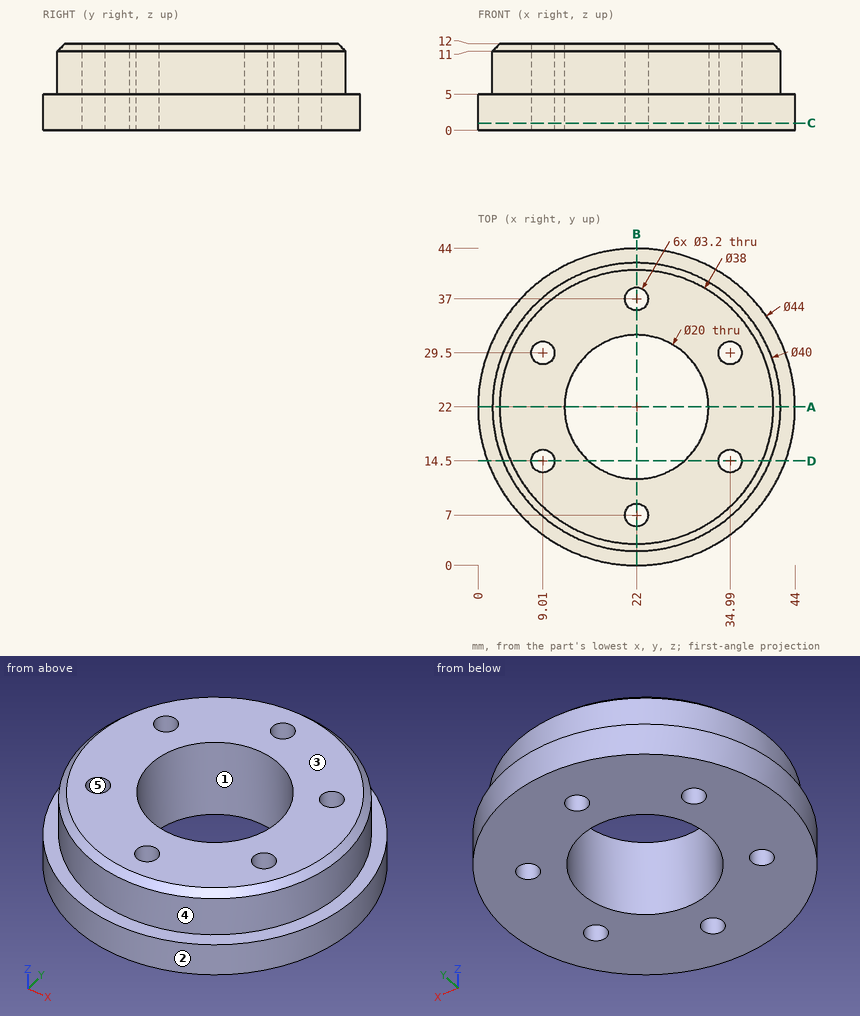
Job drawing, mm, ordinate dimensions from the low corner. One solid piece. A direction names the side the tool comes from. Round coordinates to 2 decimals unless told otherwise and drop trailing zeros. Write each loop counter-clockwise with the first axis right and the second up, starting at its lowest first coordinate (ties: lowest second). Pieces come first, ordered by that corner, then holes.
1) Mould opens along X. For the marked faces 1, 2 and 3 say: +X half, -X half, draft (parallel to the pull), parting line (faces both ways), or undercut.
2) Pin check, flat tips, straight feed: pin 1 (6 mm diameter, centred on y = 14, z = 9, fed in from +X) (1 decimal); pin 2 (3.5 mm diameter, centred on x = 34.99, y = 29.5, fed in from +Z); pin 3 (1 mm diameter, centred on y = 30.5, z = 10.5, fed in from -X); pin 4 (1.5 mm diameter, centred on y = 38, z = 10.5, fed in from -X). Stop position of each tip, or through.
3) 3-axis set-ups, long thin cutter, end or side, ignore diameter. For the marked faces 4 and 5: which of +Z, -Z, +X, -X, +Y, -Y reach the whole face in a straight line?
4) Band-saw the part on C-C, the plane z = 1. List the corners of the cut face in (x, y), and give its area (3 significant figures).
5) Band-saw the part on D-D, the plane y = 14.5. Give the number of separate pieces and of enclosed holes in the cut face, and give its area (3 significant figures).
6) Drill centre lines: probe 1 along Y at (x, z) = (22, 5.5); probe 2 along X at (y, z) = (29.5, 5.5) (1 decimal); probe 3 along Y at (x, z) = (10, 7.75) (1 decimal). Where is each one in solid material? Low to high.
7) Band-saw the part on A-A, the plane y = 22. List the corners of the cut face in (x, z), and give its area (3 significant figures).
8) Band-saw the part on B-B, the plane x = 22. List the corners of the cut face in (y, z).
Ans:
1. face 1: undercut
1. face 2: parting line
1. face 3: draft
2. pin 1: stops at x = 41.4
2. pin 2: stops at z = 12
2. pin 3: stops at x = 3.67
2. pin 4: stops at x = 9.06
3. face 4: +Z
3. face 5: +Z, -Z
4. outline: circle Ø44 at (22, 22); hole circle Ø3.2 at (9.01, 14.5); hole circle Ø3.2 at (9.01, 29.5); hole circle Ø20 at (22, 22); hole circle Ø3.2 at (22, 7); hole circle Ø3.2 at (22, 37); hole circle Ø3.2 at (34.99, 14.5); hole circle Ø3.2 at (34.99, 29.5)
4. area: 1,160 mm2
5. separate pieces: 4
5. enclosed holes: 0
5. area: 230 mm2
6. probe 1: y = 2 to 5.4, 8.6 to 12, 32 to 35.4, 38.6 to 42
6. probe 2: x = 3.5 to 7.4, 10.6 to 15.4, 28.6 to 33.4, 36.6 to 40.5
6. probe 3: y = 6 to 13.2, 15.8 to 28.2, 30.8 to 38
7. outline: (0, 0) - (12, 0) - (12, 12) - (3, 12) - (2, 11) - (2, 5) - (0, 5) - close; (32, 0) - (44, 0) - (44, 5) - (42, 5) - (42, 11) - (41, 12) - (32, 12) - close
7. area: 259 mm2
8. outline: (0, 0) - (5.4, 0) - (5.4, 12) - (3, 12) - (2, 11) - (2, 5) - (0, 5) - close; (8.6, 0) - (12, 0) - (12, 12) - (8.6, 12) - close; (32, 0) - (35.4, 0) - (35.4, 12) - (32, 12) - close; (38.6, 0) - (44, 0) - (44, 5) - (42, 5) - (42, 11) - (41, 12) - (38.6, 12) - close
